from build123d import *

# Parameters (mm, degrees)
SKETCH1_R                  = 2.286
EXTRUDE1_DEPTH             = 25.4
SKETCH2_W                  = 4.572
SKETCH2_H                  = 2.54
EXTRUDE2_DEPTH             = 7.62
SKETCH3_OUTSIDE_W          = 13.302
SKETCH3_OUTSIDE_H          = 13.302
SKETCH3_OUTSIDE_R          = 2.286
CUT_EXTRUDE1_DEPTH         = 7.62
TAP_DRILL_FOR_4_TAP1_D     = 2.2606
TAP_DRILL_FOR_4_TAP1_DEPTH = 6.35
TAP_DRILL_FOR_4_TAP1_TIP   = 0.679152758


with BuildPart() as part:
    # Sketch1 → Extrude1 (new body)
    with BuildSketch(Plane(origin=(0, 0, 0), x_dir=(1, 0, 0), z_dir=(0, 1, 0))):
        Circle(SKETCH1_R)
    extrude(amount=EXTRUDE1_DEPTH)

    # Sketch2 → Extrude2 (add)
    with BuildSketch(Plane(origin=(0, 25.4, 0), x_dir=(-1, 0, 0), z_dir=(0, 1, 0))):
        Rectangle(SKETCH2_W, SKETCH2_H)
    extrude(amount=EXTRUDE2_DEPTH)

    # Sketch3 outside → Cut-Extrude1 (cut)
    with BuildSketch(Plane(origin=(0, 25.4, 0), x_dir=(-1, 0, 0), z_dir=(0, 1, 0))):
        Rectangle(SKETCH3_OUTSIDE_W, SKETCH3_OUTSIDE_H)
        Circle(SKETCH3_OUTSIDE_R, mode=Mode.SUBTRACT)
    extrude(amount=CUT_EXTRUDE1_DEPTH, mode=Mode.SUBTRACT)

    # Tap Drill for #4 Tap1
    with Locations(Plane(origin=(-5.8e-08, 30.48, -1.27), x_dir=(-1, 0, 0), z_dir=(0, 0, -1))):
        with Locations((0, 0)):
            Hole(TAP_DRILL_FOR_4_TAP1_D / 2, depth=TAP_DRILL_FOR_4_TAP1_DEPTH)
            with Locations((0, 0, -(TAP_DRILL_FOR_4_TAP1_DEPTH + TAP_DRILL_FOR_4_TAP1_TIP / 2))):  # 118° drill point
                Cone(0, TAP_DRILL_FOR_4_TAP1_D / 2, TAP_DRILL_FOR_4_TAP1_TIP, mode=Mode.SUBTRACT)


solid = part.part
Geometry: final body of the model. Coordinates: model frame, mm. A direction names the side the tool comes from. Give positions to 0.01 mm unless a question says otherwise; leave off trailing zeros. Write each loop counter-clockwise with the first axis right and the second up, starting at its lowest first coordinate (ties: lowest second). Pieces come first, ordered by that corner, then holes. Notation, with made-up numbers: (19, -22) - (23, -22) arc R21 cw to (23, 14) - close; hole circle Ø1 at (-25, 36). An arc over 180 degrees is marked (long way). Return JSON: item names as keys, results as strings. Group by question number.
1) Section A-A on y = 30.48. Return the cut outline in (x, z), plus the area to 3 significant figures.
2) Line query: line 1 (Y direction, x = 0, z = -0.1); line 2 (X direction, y = 19.5, z = 0.15); line 3 (Y direction, x = 0.45, z = 1.9). Output: solid intervals per line, ascending.
3) Section C-C on y = 17. Return the cut outline in (x, z).
4) Set-up query: faces 3 (the flat face through (0, 0, 0)), 4 (the flat face through (0, 25.4, 2)), 5 (the flat face through (0, 25.4, -2)). Return all of +Z, -Z, +X, -X, +Y, -Y with unobstructed straight access to the full face (end or side cutting, diameter ignored); none if empty.
5) First-contact query: P1, Ø2, axis at x = 1, z = -0.5, coming from the -Y side; P2, Ø1.1, axis at x = 0.5, y = 30, coming from the +Z side; P3, Ø0.5, axis at x = -0.5, z = -2, coming from the +Y side; P4, Ø1, axis at y = 29.5, z = -1.5, coming from the +X side. Flat tips, straight axial feed; report the tip coordinate or a pass-through.
6) Mould query, pull axis X, two halves, no side actions, for faces 1 (the flat face through (0, 29, -1.27)), 2 (the cylindrical face through (0.522, 29.477, 0.018)). Classes: released by +X, released by -X, zero draft, split by the parting line, or undercut.
Filled in:
{
 "1": {"outline": "(-1.9, -1.27) - (-1.13, -1.27) - (-1.13, 1.27) - (-1.9, 1.27) arc R2.29 ccw to start; (1.13, -1.27) - (1.9, -1.27) arc R2.29 ccw to (1.9, 1.27) - (1.13, 1.27) - close", "area": "5.24 mm^2"},
 "2": {"line 1": "y = 0 to 29.35, 31.61 to 33.02", "line 2": "x = -2.28 to 2.28", "line 3": "y = 0 to 25.4"},
 "3": {"outline": "circle Ø4.57 at (0, 0)"},
 "4": {"face 3": "+Z, -Z, +X, -X, -Y", "face 4": "+Z, +X, -X, +Y", "face 5": "-Z, +X, -X, +Y"},
 "5": {"P1": "stops at y = 0", "P2": "stops at z = 1.27", "P3": "stops at y = 25.4", "P4": "stops at x = 2.06"},
 "6": {"face 1": "zero draft", "face 2": "undercut"}
}
